Here's how the part is built. I have some questions about the finished solid (model axes, mm). A direction names the side the tool comes from. Round coordinates to 2 decimals unless told otherwise and drop trailing zeros. Loops run counter-clockwise (first coordinate to the right, second up) from the corner with the lowest first, then second, coordinate; pieces in that order, holes last. Notation, with made-up numbers: (71.5, 60) - (111.5, 60) arc R23 ccw to (111.5, 92) - close; hole circle Ø6 at (16, 0). An arc over 180 degrees is marked (long way). Answer as a JSON object with one key per item and string values. Group by question number.
1) If I drill on line 1 along Z through (x, y) = (-43.18, 2.75); line 2 along X through (y, z) = (3.5, 30.48); line 3 along Z through (x, y) = (43.18, 1.2), over which ranges is the centre line in solid material (lowest first)? Write a range as [from, to].
2) Which directions (+Z, -Z, +X, -X, +Y, -Y) give clear straight access to the entire face, cutting with the end or side of a thin tool? Please do faces 1 (the face through (44.38, 2.64, 30.43)), 2 (the face through (-1, 1.588, 0)).
3) I want a section at D-D, the plane z = 12.5. Please give me the cut outline in (x, y), then the cut area to 3 significant figures.
4) If we mould it in two halves opening along Z, with no side actions, what happens to faces 3 (the face through (-1, 3, -36.83)), 4 (the face through (38.9, 0.78, 26.33)), 5 (the face through (-49.53, 3, 1))? For each: pulls with the +Z half, pulls with the -Z half, needs draft (parallel to the pull), parting line crosses it, or undercut.
5) Will these pins go through, and if not, where does the flat tip stop? P1, Ø1.5, axis at x = -9.5, z = 11.5, coming from the -Y side; P2, Ø4, axis at x = -43.18, z = -30.48, coming from the +Y side; P3, Ø2, axis at x = -43.18, z = 30.48, coming from the -Y side; P4, Ø3, axis at x = 43.18, z = -30.48, coming from the +Y side.
6) I want a section at A-A, the plane x = -43.18. Please give me the cut outline in (y, z), then the cut area to 3 significant figures.
7) I want a section at C-C, the plane x = 26. Please give me the cut outline in (y, z), then the cut area to 3 significant figures.
8) I want a section at B-B, the plane z = 30.48. Please give me the cut outline in (x, y), then the cut area to 3 significant figures.
from build123d import *

# Parameters (mm, degrees)
SKETCH1_W                                       = 99.06
SKETCH1_H                                       = 73.66
BOSS_EXTRUDE1_DEPTH                             = 6.35
CSK_FOR_M2_FLAT_HEAD_MACHINE_SCREW1_D           = 2.4
CSK_FOR_M2_FLAT_HEAD_MACHINE_SCREW1_CSINK_D     = 4.4
CSK_FOR_M2_FLAT_HEAD_MACHINE_SCREW1_CSINK_ANGLE = 90
SHELL1_DEPTH                                    = 1.5875


# Read off the part's stored shape, not the designer's step: Shell1
with BuildPart() as part:
    # Sketch1 → Boss-Extrude1 (new body)
    with BuildSketch(Plane(origin=(0, 0, 0), x_dir=(1, 0, 0), z_dir=(0, 1, 0))):
        Rectangle(SKETCH1_W, SKETCH1_H)
    extrude(amount=BOSS_EXTRUDE1_DEPTH)

    # CSK for M2 Flat Head Machine Screw1 (through all)
    with Locations(Plane(origin=(0, 6.35, 0), x_dir=(1, 0, 0), z_dir=(0, 1, 0))):
        with Locations((-43.18, 30.48), (-43.18, -30.48), (43.18, -30.48), (43.18, 30.48)):
            CounterSinkHole(CSK_FOR_M2_FLAT_HEAD_MACHINE_SCREW1_D / 2, CSK_FOR_M2_FLAT_HEAD_MACHINE_SCREW1_CSINK_D / 2, counter_sink_angle=CSK_FOR_M2_FLAT_HEAD_MACHINE_SCREW1_CSINK_ANGLE)

    # Shell1 outline → Shell1 (cut)
    with BuildSketch(Plane(origin=(0, 0, 0), x_dir=(1, 0, 0), z_dir=(0, 1, 0))):
        with BuildLine():
            Line((44.7675, -24.732718034), (44.7675, 24.732718034))
            ThreePointArc((44.7675, 24.732718034), (38.963875817, 26.263875817), (37.432718034, 32.0675))
            Line((37.432718034, 32.0675), (-37.432718034, 32.0675))
            ThreePointArc((-37.432718034, 32.0675), (-38.963875817, 26.263875817), (-44.7675, 24.732718034))
            Line((-44.7675, 24.732718034), (-44.7675, -24.732718034))
            ThreePointArc((-44.7675, -24.732718034), (-38.963875817, -26.263875817), (-37.432718034, -32.0675))
            Line((-37.432718034, -32.0675), (37.432718034, -32.0675))
            ThreePointArc((37.432718034, -32.0675), (38.963875817, -26.263875817), (44.7675, -24.732718034))
        make_face()
    extrude(amount=SHELL1_DEPTH, mode=Mode.SUBTRACT)


solid = part.part
Outcome:
{
 "1": {"line 1": "[-36.83, -31.68], [-29.28, 29.28], [31.68, 36.83]", "line 2": "[-49.53, -44.38], [-41.98, 41.98], [44.38, 49.53]", "line 3": "[-36.83, -31.68], [-29.28, -24.52], [24.52, 29.28], [31.68, 36.83]"},
 "2": {"face 1": "+Y, -Y", "face 2": "-Y"},
 "3": {"outline": "(-49.53, 0) - (-44.77, 0) - (-44.77, 1.59) - (44.77, 1.59) - (44.77, 0) - (49.53, 0) - (49.53, 6.35) - (-49.53, 6.35) - close", "area": "487 mm^2"},
 "4": {"face 3": "pulls with the -Z half", "face 4": "undercut", "face 5": "needs draft"},
 "5": {"P1": "y = 1.59", "P2": "y = 6.15", "P3": "through", "P4": "y = 5.65"},
 "6": {"outline": "(0, -36.83) - (6.35, -36.83) - (6.35, -32.68) - (5.35, -31.68) - (0, -31.68) - close; (0, -29.28) - (5.35, -29.28) - (6.35, -28.28) - (6.35, 28.28) - (5.35, 29.28) - (0, 29.28) - (0, 24.52) - (1.59, 24.52) - (1.59, -24.52) - (0, -24.52) - close; (0, 31.68) - (5.35, 31.68) - (6.35, 32.68) - (6.35, 36.83) - (0, 36.83) - close", "area": "357 mm^2"},
 "7": {"outline": "(0, -36.83) - (6.35, -36.83) - (6.35, 36.83) - (0, 36.83) - (0, 32.07) - (1.59, 32.07) - (1.59, -32.07) - (0, -32.07) - close", "area": "366 mm^2"},
 "8": {"outline": "(-49.53, 0) - (-44.38, 0) - (-44.38, 5.35) - (-45.38, 6.35) - (-49.53, 6.35) - close; (-41.98, 0) - (-37.22, 0) - (-37.22, 1.59) - (37.22, 1.59) - (37.22, 0) - (41.98, 0) - (41.98, 5.35) - (40.98, 6.35) - (-40.98, 6.35) - (-41.98, 5.35) - close; (44.38, 0) - (49.53, 0) - (49.53, 6.35) - (45.38, 6.35) - (44.38, 5.35) - close", "area": "478 mm^2"}
}
